```python
from build123d import *

# Parameters (mm, degrees)
SKETCH1_W           = 40.4
SKETCH1_H           = 26
SKETCH1_W_2         = 34.4
SKETCH1_H_2         = 20.4
BOSS_EXTRUDE1_DEPTH = 22
SKETCH2_W           = 40.4
SKETCH2_H           = 26
BOSS_EXTRUDE2_DEPTH = 1.4
SKETCH3_W           = 12.5
SKETCH3_H           = 8
CUT_EXTRUDE1_DEPTH  = 15
SKETCH4_R           = 1.2
CUT_EXTRUDE2_DEPTH  = 24.4
SKETCH5_W           = 10
SKETCH5_H           = 6
BOSS_EXTRUDE3_DEPTH = 23.4
FILLET1_R           = 2
SKETCH6_R           = 1.65
CUT_EXTRUDE3_DEPTH  = 7
CHAMFER1_SIZE       = 1
SKETCH8_W           = 4
SKETCH8_H           = 8
CUT_EXTRUDE4_DEPTH  = 4
CHAMFER2_SIZE       = 1
SKETCH9_R           = 3.2
SKETCH9_R_2         = 1.2
BOSS_EXTRUDE4_DEPTH = 0.6


with BuildPart() as part:
    # Sketch1 → Boss-Extrude1 (new body)
    with BuildSketch(Plane.XY):
        Rectangle(SKETCH1_W, SKETCH1_H)
        Rectangle(SKETCH1_W_2, SKETCH1_H_2, mode=Mode.SUBTRACT)
    extrude(amount=BOSS_EXTRUDE1_DEPTH)

    # Sketch2 → Boss-Extrude2 (add)
    with BuildSketch(Plane.XY.offset(22)):
        Rectangle(SKETCH2_W, SKETCH2_H)
    extrude(amount=BOSS_EXTRUDE2_DEPTH)

    # Sketch3 → Cut-Extrude1 (cut)
    with BuildSketch(Plane.XY.offset(23.4)):
        with Locations((-1.7, 9)):
            Rectangle(SKETCH3_W, SKETCH3_H)
        with Locations((-1.7, -9)):
            Rectangle(SKETCH3_W, SKETCH3_H)
    extrude(amount=-CUT_EXTRUDE1_DEPTH, mode=Mode.SUBTRACT)

    # Sketch4 → Cut-Extrude2 (cut, through all)
    with BuildSketch(Plane.XY.offset(23.4)):
        with Locations((-15, 8)):
            Circle(SKETCH4_R)
        with Locations((-15, -8)):
            Circle(SKETCH4_R)
        with Locations((15, 8)):
            Circle(SKETCH4_R)
        with Locations((15, -8)):
            Circle(SKETCH4_R)
    extrude(amount=-CUT_EXTRUDE2_DEPTH, mode=Mode.SUBTRACT)

    # Sketch5 → Boss-Extrude3 (add)
    with BuildSketch(Plane(origin=(0, 0, 0), x_dir=(-1, 0, 0), z_dir=(0, 0, -1))):
        with Locations((-25.2, -10)):
            Rectangle(SKETCH5_W, SKETCH5_H)
        with Locations((25.2, -10)):
            Rectangle(SKETCH5_W, SKETCH5_H)
    extrude(amount=-BOSS_EXTRUDE3_DEPTH)

    # Fillet1
    fillet1_edges = [part.edges().sort_by_distance(p)[0] for p in [
        (30.2, -10, 0),
        (30.2, -10, 23.4),
        (20.2, -7, 11.7),
        (-30.2, -10, 0),
        (-30.2, -10, 23.4),
        (-20.2, -7, 11.7),
        (-20.2, 13, 11.7),
        (20.2, 13, 11.7),
    ]]
    fillet(fillet1_edges, radius=FILLET1_R)

    # Sketch6 → Cut-Extrude3 (cut, through all)
    with BuildSketch(Plane(origin=(0, -7, 0), x_dir=(1, 0, 0), z_dir=(0, 1, 0))):
        with Locations((26.2, -4.2)):
            Circle(SKETCH6_R)
        with Locations((26.2, -19.2)):
            Circle(SKETCH6_R)
        with Locations((-26.2, -19.2)):
            Circle(SKETCH6_R)
        with Locations((-26.2, -4.2)):
            Circle(SKETCH6_R)
    extrude(amount=-CUT_EXTRUDE3_DEPTH, mode=Mode.SUBTRACT)

    # Chamfer1
    chamfer1_edges = [part.edges().sort_by_distance(p)[0] for p in [
        (-27.85, -7, 4.2),
        (-27.85, -7, 19.2),
        (24.55, -7, 19.2),
        (24.55, -7, 4.2),
    ]]
    chamfer(chamfer1_edges, length=CHAMFER1_SIZE)

    # Sketch8 → Cut-Extrude4 (cut)
    with BuildSketch(Plane.XY.offset(23.4)):
        with Locations((18.2, 0)):
            Rectangle(SKETCH8_W, SKETCH8_H)
    extrude(amount=-CUT_EXTRUDE4_DEPTH, mode=Mode.SUBTRACT)

    # Chamfer2
    chamfer2_edges = [part.edges().sort_by_distance(p)[0] for p in [
        (16.2, -4, 22.7),
        (16.2, 4, 22.7),
        (18.7, 4, 19.4),
        (18.7, -4, 19.4),
    ]]
    chamfer(chamfer2_edges, length=CHAMFER2_SIZE)

    # Sketch9 → Boss-Extrude4 (add)
    with BuildSketch(Plane.XY.offset(23.4)):
        with Locations((-15, 8)):
            Circle(SKETCH9_R)
        with Locations((-15, 8)):
            Circle(SKETCH9_R_2, mode=Mode.SUBTRACT)
        with Locations((-15, -8)):
            Circle(SKETCH9_R)
        with Locations((-15, -8)):
            Circle(SKETCH9_R_2, mode=Mode.SUBTRACT)
        with Locations((15, -8)):
            Circle(SKETCH9_R)
        with Locations((15, -8)):
            Circle(SKETCH9_R_2, mode=Mode.SUBTRACT)
        with Locations((15, 8)):
            Circle(SKETCH9_R)
        with Locations((15, 8)):
            Circle(SKETCH9_R_2, mode=Mode.SUBTRACT)
    extrude(amount=BOSS_EXTRUDE4_DEPTH)


solid = part.part
```
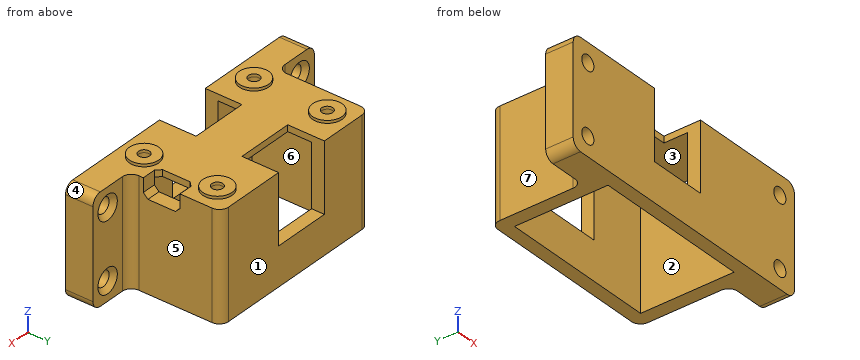
Source: CAD feature listing. Evaluate the final solid. Frame: model axes, mm. Face numbers are marked on the shaded views. A direction names the side the tool comes from. Round coordinates to 2 decimals unless told otherwise and drop trailing zeros. Loops run counter-clockwise (first coordinate to the right, second up) from the corner with the lowest first, then second, coordinate; pieces in that order, holes last. Notation, with made-up numbers: (70, 84) - (127, 84) arc R8 cw to (127, 94) - close; hole circle Ø4 at (86.25, 53.5). An arc over 180 degrees is marked (long way). Use CSV: the item, a comma, the result in double quotes.
Q1. Section query A-A, the plane x = -26.2. Output: boundary loops of the cut face in (y, z).
Reported:
outline,"(-13, 0) - (-7, 0) - (-7, 1.55) - (-8, 2.55) - (-13, 2.55) - close; (-13, 5.85) - (-8, 5.85) - (-7, 6.85) - (-7, 16.55) - (-8, 17.55) - (-13, 17.55) - close; (-13, 20.85) - (-8, 20.85) - (-7, 21.85) - (-7, 23.4) - (-13, 23.4) - close"
Q2. Reachability of the marked faces 5, 6 and 7 from +Z, -Z, +X, -X, +Y, -Y: full face, straight path, thin tool, end or side. Return the list, or none.
Reported:
face 5,"+Z, -Z, +X, +Y"
face 6,"-Z"
face 7,"+Z, -Z, -X, +Y"
Q3. Ray query, line 1 along Y through (x, z) = (-15, 22.8); line 2 along Y through (x, z) = (-15, 23.6); line 3 along X through (y, z) = (2, 11.75). Return the intervals inside material, ascending.
Reported:
line 1,"-13 to -9.2, -6.8 to 6.8, 9.2 to 13"
line 2,"-11.2 to -9.2, -6.8 to -4.8, 4.8 to 6.8, 9.2 to 11.2"
line 3,"-20.2 to -17.2, 17.2 to 20.2"
Q4. Section query C-C, the plane z = 12. Output: boundary loops of the cut face in (x, y).
Reported:
outline,"(-30.2, -13) - (-7.95, -13) - (-7.95, -10.2) - (-17.2, -10.2) - (-17.2, 10.2) - (-7.95, 10.2) - (-7.95, 13) - (-18.2, 13) arc R2 ccw to (-20.2, 11) - (-20.2, -5) arc R2 cw to (-22.2, -7) - (-30.2, -7) - close; (4.55, -13) - (30.2, -13) - (30.2, -7) - (22.2, -7) arc R2 cw to (20.2, -5) - (20.2, 11) arc R2 ccw to (18.2, 13) - (4.55, 13) - (4.55, 10.2) - (17.2, 10.2) - (17.2, -10.2) - (4.55, -10.2) - close"
Q5. Section query B-B, the plane z = 4.2. Output: boundary loops of the cut face in (x, y), then the cut area to 3 significant figures.
Reported:
outline,"(-30.2, -13) - (-27.85, -13) - (-27.85, -8) - (-28.85, -7) - (-30.2, -7) - close; (-24.55, -13) - (24.55, -13) - (24.55, -8) - (23.55, -7) - (22.2, -7) arc R2 cw to (20.2, -5) - (20.2, 11) arc R2 ccw to (18.2, 13) - (-18.2, 13) arc R2 ccw to (-20.2, 11) - (-20.2, -5) arc R2 cw to (-22.2, -7) - (-23.55, -7) - (-24.55, -8) - close; (27.85, -13) - (30.2, -13) - (30.2, -7) - (28.85, -7) - (27.85, -8) - close; hole (-17.2, -10.2) - (17.2, -10.2) - (17.2, 10.2) - (-17.2, 10.2) - close"
area,"427 mm^2"
Q6. Pin query (flat end, axial travel): pin 1 Ø5 at (y, z) = (1.5, 10.5) entering from -X; pin 2 Ø2 at (x, z) = (23, 10.5) entering from +Y; pin 3 Ø12 at (x, y) = (2.5, 1.5) entering from +Z; pin 4 Ø1.4 at (x, y) = (15, -8) entering from +Z. Return the tip coordinate at first contact, or that it passes through.
Reported:
pin 1,"x = -20.2"
pin 2,"y = -6.99"
pin 3,"z = 23.4"
pin 4,"through"
Q7. Mould query, pull axis Y, two halves, no side actions, for the marked faces 1, 2, 3 and 4. Classes: pulls with the +Y half, pulls with the -Y half, needs draft (parallel to the pull), parting line crosses it, or undercut.
Reported:
face 1,"pulls with the +Y half"
face 2,"undercut"
face 3,"undercut"
face 4,"needs draft"
Q8. Section query D-D, the plane y = 2. Output: boundary loops of the cut face in (x, z).
Reported:
outline,"(-20.2, 0) - (-17.2, 0) - (-17.2, 22) - (16.2, 22) - (16.2, 23.4) - (-20.2, 23.4) - close; (17.2, 0) - (20.2, 0) - (20.2, 19.4) - (17.2, 19.4) - close"
